For this review, take the finished solid that the model builds, in its own axes (mm). Give positions to 0.01 mm unless a question says otherwise; leave off trailing zeros. Write each loop counter-clockwise with the first axis right and the second up, starting at its lowest first coordinate (ties: lowest second). Pieces come first, ordered by that corner, then holes.
1) We need section B-B on z = 69. Give the boundary of the cut face in (x, y), and give its area (3 significant figures).
2) We need section C-C on y = 137. Give the boundary of the cut face in (x, z).
3) Draft analysis for pull direction X (two halves, no side actions). For faces 1 (the face through (-1.416, 126.289, 16.514)), 2 (the face through (-1.377, 126.289, 8.906)), 3 (the face through (-2.794, 126, 13)), 4 (the face through (1, 139, 101.6)), state which applies: pulls with the +X half, pulls with the -X half, needs draft (parallel to the pull), parting line crosses it, or undercut.
4) For P1, Ø8, axis at y = 132, z = 65, coming from the -X side; P2, Ø1, axis at y = 135, z = 52.5, coming from the +X side; P3, Ø0.8, axis at x = -1.5, z = 14.5, coming from the -Y side, all flat-tipped, find the tip position at first contact; note any pin that passes through.
5) We need section A-A on y = 147.5. Give the boundary of the cut face in (x, z), and give its area (3 significant figures).
6) Wall thickness on line 1 along X through (y, z) = (163.5, 16.5); line 2 along Z through (x, y) = (-1.25, 154); line 3 along Z through (x, y) = (4, 120): over which ranges is each line inside the solid? List them lowest first.
from build123d import *

# Parameters (mm, degrees)
BOSS_EXTRUDE1_DEPTH      = 101.6
BOSS_EXTRUDE2_REACH      = 145.703
BOSS_EXTRUDE2_END_RADIUS = 177.8
BOSS_EXTRUDE3_REACH      = 145.805
BOSS_EXTRUDE3_END_RADIUS = 177.8


with BuildPart() as part:
    # Sketch1 → Boss-Extrude1 (new body)
    with BuildSketch(Plane.XY):
        with BuildLine():
            Line((0, 76.2), (0, 177.8))
            ThreePointArc((0, 177.8), (1.551578012, 177.793229921), (3.103037865, 177.772920199))
            Line((3.103037865, 177.772920199), (1.329873371, 76.188394371))
            ThreePointArc((1.329873371, 76.188394371), (0.664962005, 76.197098537), (0, 76.2))
        make_face()
    extrude(amount=BOSS_EXTRUDE1_DEPTH)

    # Boss-Extrude2: up to this cylinder (the profile starts inside it)
    boss_extrude2_end = Plane(origin=(0, 0, 50.8), z_dir=(0, 0, -1)) * Cylinder(BOSS_EXTRUDE2_END_RADIUS, 724.206, mode=Mode.PRIVATE)
    # Sketch2 → Boss-Extrude2 (add, up to the surface)
    with BuildSketch(Plane(origin=(1.329873371, 76.188394371, 0), x_dir=(0, 0, -1), z_dir=(-0.01745240643728355, -0.9998476951563914, 0)), mode=Mode.PRIVATE) as boss_extrude2_sk1:
        Polygon((-92.000208065, 0), (-93.4085, 2.794), (-84.3915, 2.794), (-85.799791935, 0), align=None)
    boss_extrude2_tool1 = extrude(boss_extrude2_sk1.sketch, amount=-BOSS_EXTRUDE2_REACH, mode=Mode.PRIVATE) & boss_extrude2_end
    add(boss_extrude2_tool1.solids().sort_by_distance((2.812837, 76.162509, 88.9))[0])
    # Sketch2 → Boss-Extrude2 (add, up to the surface)
    with BuildSketch(Plane(origin=(1.329873371, 76.188394371, 0), x_dir=(0, 0, -1), z_dir=(-0.01745240643728355, -0.9998476951563914, 0)), mode=Mode.PRIVATE) as boss_extrude2_sk2:
        Polygon((-15.800208065, 0), (-9.599791935, 0), (-8.1915, 2.794), (-17.2085, 2.794), align=None)
    boss_extrude2_tool2 = extrude(boss_extrude2_sk2.sketch, amount=-BOSS_EXTRUDE2_REACH, mode=Mode.PRIVATE) & boss_extrude2_end
    add(boss_extrude2_tool2.solids().sort_by_distance((2.812837, 76.162509, 12.7))[0])

    # Boss-Extrude3: up to this cylinder (the profile starts inside it)
    boss_extrude3_end = Plane(origin=(0, 0, 50.8), z_dir=(0, 0, -1)) * Cylinder(BOSS_EXTRUDE3_END_RADIUS, 724.41, mode=Mode.PRIVATE)
    # Sketch3 → Boss-Extrude3 (add, up to the surface)
    with BuildSketch(Plane(origin=(0, 76.2, 0), x_dir=(0, 0, -1), z_dir=(0, -1, 0)), mode=Mode.PRIVATE) as boss_extrude3_sk1:
        Polygon((-92.000208065, 0), (-93.4085, -2.79357446), (-84.3915, -2.79357446), (-85.799791935, 0), align=None)
    boss_extrude3_tool1 = extrude(boss_extrude3_sk1.sketch, amount=-BOSS_EXTRUDE3_REACH, mode=Mode.PRIVATE) & boss_extrude3_end
    add(boss_extrude3_tool1.solids().sort_by_distance((-1.482964, 76.2, 88.9))[0])
    # Sketch3 → Boss-Extrude3 (add, up to the surface)
    with BuildSketch(Plane(origin=(0, 76.2, 0), x_dir=(0, 0, -1), z_dir=(0, -1, 0)), mode=Mode.PRIVATE) as boss_extrude3_sk2:
        Polygon((-15.800208065, 0), (-9.599791935, 0), (-8.1915, -2.79357446), (-17.2085, -2.79357446), align=None)
    boss_extrude3_tool2 = extrude(boss_extrude3_sk2.sketch, amount=-BOSS_EXTRUDE3_REACH, mode=Mode.PRIVATE) & boss_extrude3_end
    add(boss_extrude3_tool2.solids().sort_by_distance((-1.482964, 76.2, 12.7))[0])


solid = part.part
Results list:
1. outline: (0, 76.2) arc R76.2 cw to (1.33, 76.19) - (3.1, 177.77) arc R177.8 ccw to (0, 177.8) - close
1. area: 225 mm2
2. outline: (-2.79, 8.19) - (0, 9.6) - (0, 0) - (2.39, 0) - (2.39, 9.6) - (5.19, 8.19) - (5.19, 17.21) - (2.39, 15.8) - (2.39, 85.8) - (5.19, 84.39) - (5.19, 93.41) - (2.39, 92) - (2.39, 101.6) - (0, 101.6) - (0, 92) - (-2.79, 93.41) - (-2.79, 84.39) - (0, 85.8) - (0, 15.8) - (-2.79, 17.21) - close
3. face 1: undercut
3. face 2: undercut
3. face 3: pulls with the -X half
3. face 4: needs draft
4. P1: stops at x = 0
4. P2: stops at x = 2.37
4. P3: stops at y = 76.2
5. outline: (-2.79, 8.19) - (0, 9.6) - (0, 0) - (2.57, 0) - (2.57, 9.6) - (5.37, 8.19) - (5.37, 17.21) - (2.57, 15.8) - (2.57, 85.8) - (5.37, 84.39) - (5.37, 93.41) - (2.57, 92) - (2.57, 101.6) - (0, 101.6) - (0, 92) - (-2.79, 93.41) - (-2.79, 84.39) - (0, 85.8) - (0, 15.8) - (-2.79, 17.21) - close
5. area: 347 mm2
6. line 1: x = -2.79 to -1.39, 0 to 2.85, 4.24 to 5.65
6. line 2: z = 8.97 to 16.43, 85.17 to 92.63
6. line 3: z = 8.64 to 16.76, 84.84 to 92.96
